Geometry check sheet. Reference: the model listing, model coordinates, mm. A direction names the side the tool comes from. Coordinates: 2 decimals unless noted, no trailing zeros. Loops run counter-clockwise (first coordinate to the right, second up) from the corner with the lowest first, then second, coordinate; pieces in that order, holes last. Notation, with made-up numbers: M 58.5,88.5 L 77.5,88.5 A23 cw 77.5,119.5 Z; hole C -36,-33.5 d10. An arc over 180 degrees is marked long. Use CSV: the item, a comma, the result in double quotes.
```python
from build123d import *

# Parameters (mm, degrees)
ESBO_O1_R                = 3
RESSALTO_EXTRUS_O1_DEPTH = 10
ESBO_O2_W                = 6
ESBO_O2_H                = 3
RESSALTO_EXTRUS_O2_DEPTH = 10


with BuildPart() as part:
    # Esboço1 → Ressalto-extrusão1 (new body)
    with BuildSketch(Plane(origin=(0, 0, 0), x_dir=(1, 0, 0), z_dir=(0, 1, 0))):
        Circle(ESBO_O1_R)
    extrude(amount=RESSALTO_EXTRUS_O1_DEPTH)

    # Esboço2 → Ressalto-extrusão2 (add)
    with BuildSketch(Plane.XZ):
        with Locations((0, 1.5)):
            Rectangle(ESBO_O2_W, ESBO_O2_H)
    extrude(amount=RESSALTO_EXTRUS_O2_DEPTH)


solid = part.part
```
1. Section check B-B, the plane z = 0.95. Record the cut outline in (x, y), plus the area to 3 significant figures.
The answers:
outline,"M -3,-10 L 3,-10 L 3,0 L 2.85,0 L 2.85,10 L -2.85,10 L -2.85,0 L -3,0 Z"
area,"117 mm^2"
2. Thickness scan on line 1 (Z direction, x = 0, y = -2.75); line 2 (Y direction, x = -0.55, z = -0.9); line 3 (Z direction, x = -2.15, y = 7). Record the ranges inside material, lowest first. Write a range as [from, to].
The answers:
line 1,"[0, 3]"
line 2,"[0, 10]"
line 3,"[-2.09, 2.09]"
3. Set-up check for faces 1 (the cylindrical face through (-3, 5, 0)), 2 (the flat face through (0, 0, -1)), 3 (the flat face through (2.3, 0, 2.4)), 4 (the flat face through (-2.4, 0, 2.3)): record each of +Z, -Z, +X, -X, +Y, -Y from which the full face is reachable in a straight line by a thin tool's end or side.
The answers:
face 1,"+Y"
face 2,"-Z, +X, -X, -Y"
face 3,"+Z, +X, +Y"
face 4,"+Z, -X, +Y"
4. Gauge pin test, flat ends, axial feed: P1, Ø3, axis at x = 1.5, z = -2, coming from the -Y side; P2, Ø1.8, axis at x = 1, y = -6, coming from the -Z side. Record the tip position at first contact, or that the pin passes through.
The answers:
P1,"y = 0"
P2,"z = 0"
5. Section check D-D, the plane y = -6.5. Record the cut outline in (x, z).
The answers:
outline,"M -3,0 L 3,0 L 3,3 L -3,3 Z"
6. Section check C-C, the plane y = 6.5. Record the cut outline in (x, z).
The answers:
outline,"C 0,0 d6"
